Design review of the part shown in the three views and the two pictorial views. Dimensions are in mm from the part's minimum x, y and z. Coordinates: 2 decimals unless noted, no trailing zeros. Order: outer loops, then holes, each group sorted by start corner. A loop starts at its lowest first (then second) coordinate and runs counter-clockwise, first axis right, second up. Notation, with made-up numbers: (8.5, -13.75) -> (56.5, -13.75) arc R23 cw to (56.5, -3.75) -> close; hole circle Ø1 at (88, 60). An arc over 180 degrees is marked (long way). Write item = value, one per line. Start each with the question number.
1) Insertion check: pin 1 Ø5 at (y, z) = (34.5, 53) entering from +X; pin 2 Ø3 at (x, y) = (99, 22.5) entering from -Z; pin 3 Ø5 at (x, y) = (33, 30.5) entering from -Z. Each pin has a flat end and moves straight along its axis. Give the tip position at first contact, or say it passes through.
2) Consider section B-B on y = 41. Give the boundary of the cut face in (x, z), and give its area (3 significant figures).
3) Wall thickness on probe 1 along Z at (x, y) = (30.5, 36.5) (1 decimal); probe 2 along X at (y, z) = (22.5, 62); probe 3 along X at (y, z) = (23.5, 109) (1 decimal): over which ranges is each line inside the solid? List them lowest first. Write a range as [from, to].
4) Consider section A-A on y = 50.5. Give the boundary of the cut face in (x, z).
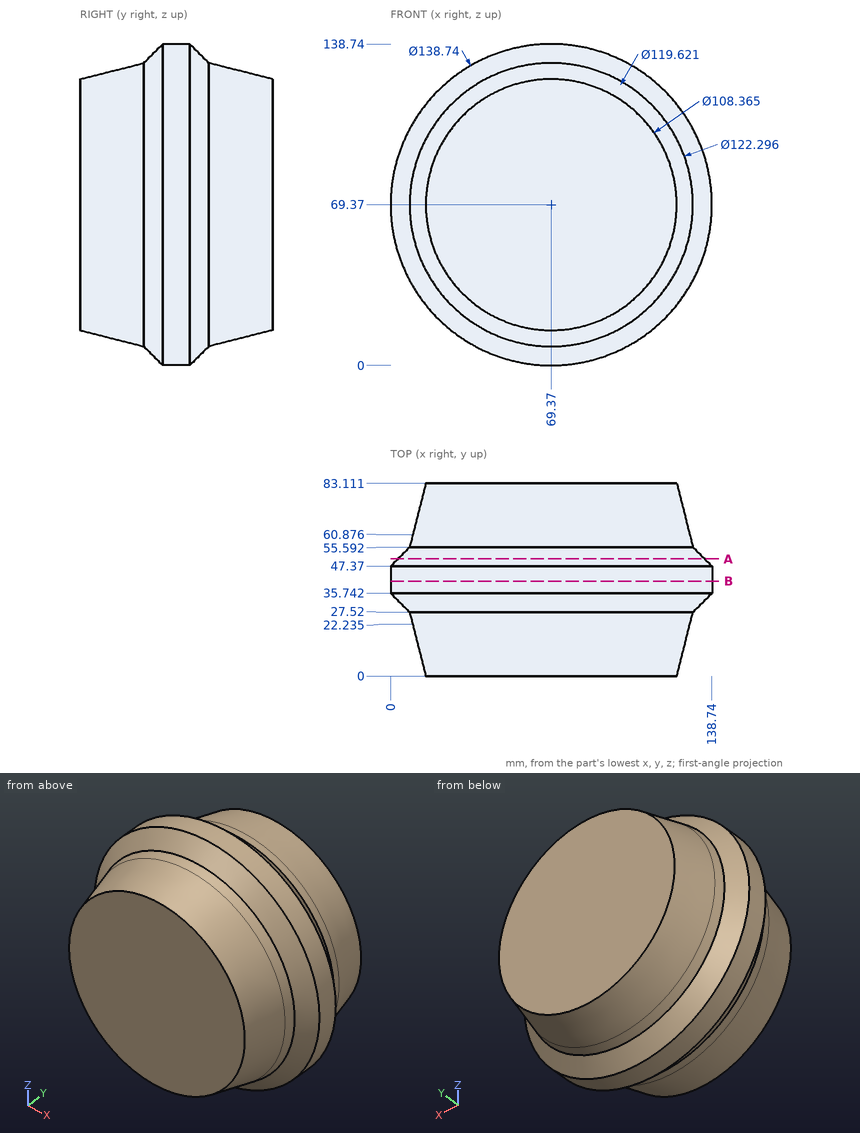
Answer sheet:
q1.pin_1 = 137.27
q1.pin_2 = 16.4
q1.pin_3 = 13.14
q2.outline = circle Ø138.74 at (69.37, 69.37)
q2.area = 15,100 mm2
q3.probe_1 = [11.9, 126.8]
q3.probe_2 = [9.95, 128.79]
q3.probe_3 = [24.1, 114.6]
q4.outline = circle Ø132.48 at (69.37, 69.37)
